Geometry: final body of the model. Coordinates: model frame, mm. Face numbers are marked on the shaded views. A direction names the side the tool comes from. Give positions to 0.01 mm unless a question says otherwise; leave off trailing zeros. Order: outer loops, then holes, each group sorted by start corner. A loop starts at its lowest first (then second) coordinate and runs counter-clockwise, first axis right, second up. Notation, with made-up numbers: (4, 17) -> (19, 17) arc R23 ccw to (19, 35) -> close; hole circle Ø6 at (83, 80). An arc over 180 degrees is marked (long way). Write item = value, one per line.
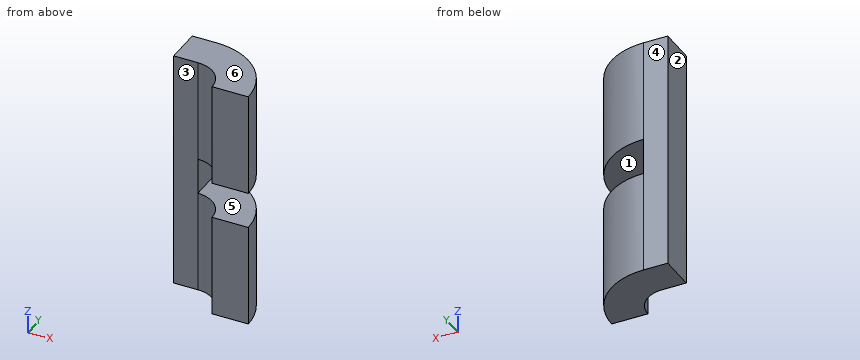
```python
from build123d import *

# Parameters (mm, degrees)
SKETCH_1_W          = 20
SKETCH_1_H          = 30
EXTRUDE_1_DEPTH     = 200
EXTRUDE_2_DEPTH     = 200
SKETCH_2_W          = 30
SKETCH_2_H          = 79.389115132
CUT_EXTRUDE_1_DEPTH = 54


with BuildPart() as part:
    # Sketch 1 → Extrude 1 (new body)
    with BuildSketch(Plane.XY):
        with Locations((10, 15)):
            Rectangle(SKETCH_1_W, SKETCH_1_H)
    extrude(amount=EXTRUDE_1_DEPTH)

    # Sketch 1_3 → Extrude 2 (add)
    with BuildSketch(Plane.XY):
        with BuildLine():
            Line((20, 0), (20, 30))
            ThreePointArc((20, 30), (58.183766184, 14.183766184), (74, -24))
            Line((74, -24), (44, -24))
            ThreePointArc((44, -24), (36.970562748, -7.029437252), (20, 0))
        make_face()
    extrude(amount=EXTRUDE_2_DEPTH)

    # Sketch 2 → Cut-Extrude 1 (cut)
    with BuildSketch(Plane(origin=(74, 0, 0), x_dir=(0, 0, -1), z_dir=(1, 0, 0))):
        with Locations((-100, 15.694557566)):
            Rectangle(SKETCH_2_W, SKETCH_2_H)
    extrude(amount=-CUT_EXTRUDE_1_DEPTH, mode=Mode.SUBTRACT)


solid = part.part
```
1) Section query C-C (z = 82.5). Output: boundary loops of the cut face in (x, y).
Check sheet entries:
outline = (0, 0) -> (20, 0) arc R24 cw to (44, -24) -> (74, -24) arc R54 ccw to (20, 30) -> (0, 30) -> close
2) Line query: line 1 (Z direction, x = 37, y = 14.5); line 2 (Y direction, x = 12.5, z = 137.5); line 3 (Y direction, x = 36, z = 65). Output: solid intervals per line, ascending. Write a range as from..to.
Check sheet entries:
line_1 = 0..85, 115..200
line_2 = 0..30
line_3 = -6.11..27.58
3) Section query A-A (y = -19.5). Output: boundary loops of the cut face in (x, z), plus the area to 3 significant figures.
Check sheet entries:
outline = (43.57, 0) -> (73.81, 0) -> (73.81, 85) -> (43.57, 85) -> close; (43.57, 115) -> (73.81, 115) -> (73.81, 200) -> (43.57, 200) -> close
area = 5,140 mm²
4) First-contact query: P1, Ø2, axis at y = 2.5, z = 124, coming from the +X side; P2, Ø3, axis at x = 43.5, z = 151.5, coming from the +Y side; P3, Ø10, axis at y = 15.5, z = 141.5, coming from the +X side; P4, Ø12, axis at x = 64.5, y = 7, coming from the +Z side. Flat tips, straight axial feed; report the tip coordinate or a pass-through.
Check sheet entries:
P1 = 67.6
P2 = 25.32
P3 = 61.54
P4 = 200
5) Mould query, pull axis Z, two halves, no side actions, for the marked faces 4, 5 and 6. Classes: +Z half, -Z half, draft (parallel to the pull), parting line (faces both ways), or undercut.
Check sheet entries:
face_4 = draft
face_5 = undercut
face_6 = +Z half
6) Section query D-D (y = 23). Output: boundary loops of the cut face in (x, z), plus the area to 3 significant figures.
Check sheet entries:
outline = (0, 0) -> (46.59, 0) -> (46.59, 85) -> (20, 85) -> (20, 115) -> (46.59, 115) -> (46.59, 200) -> (0, 200) -> close
area = 8,520 mm²
7) Section query B-B (x = 24). Output: boundary loops of the cut face in (y, z).
Check sheet entries:
outline = (-0.34, 0) -> (29.85, 0) -> (29.85, 85) -> (-0.34, 85) -> close; (-0.34, 115) -> (29.85, 115) -> (29.85, 200) -> (-0.34, 200) -> close
8) Reachability of the marked faces 1, 2 and 3 from +Z, -Z, +X, -X, +Y, -Y: full face, straight path, thin tool, end or side. Return the list, or none.
Check sheet entries:
face_1 = +X, +Y, -Y
face_2 = +Z, -Z, -X, +Y, -Y
face_3 = +Z, -Z, -X, -Y
